Here's how the part is built. I have some questions about the finished solid (model axes, mm). Face numbers are marked on the shaded views. Give positions to 0.01 mm unless a question says otherwise; leave off trailing zeros. Order: outer loops, then holes, each group sorted by start corner. A loop starts at its lowest first (then second) coordinate and runs counter-clockwise, first axis right, second up. Notation, with made-up numbers: M -19,22 L -5,22 A23 ccw -5,48 Z; hole C -7,80 d4. An arc over 180 degrees is marked long. Use one line per item in the form item = value.
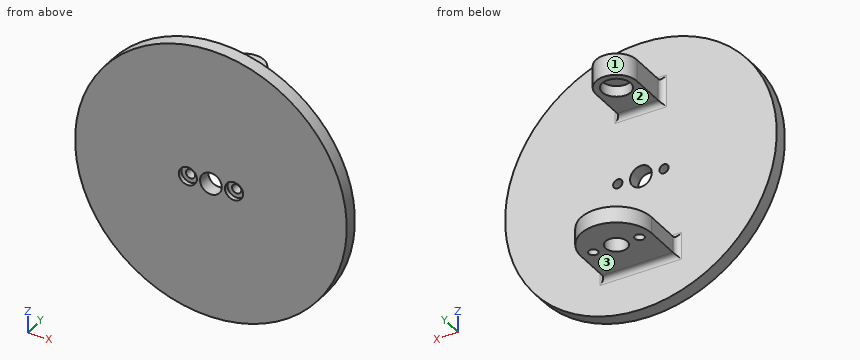
from build123d import *

# Parameters (mm, degrees)
SKETCH1_R                       = 50
SKETCH1_R_2                     = 4
BOSS_EXTRUDE1_DEPTH             = 5
BOSS_EXTRUDE4_DEPTH             = 6
BOSS_EXTRUDE5_DEPTH             = 8
CBORE_FOR_M3_SBHCS1_D           = 3.4
CBORE_FOR_M3_SBHCS1_CBORE_D     = 6.7
CBORE_FOR_M3_SBHCS1_CBORE_DEPTH = 1.65
CBORE_START                     = -29.65
CBORE_FOR_M3_SBHCS2_OUTLINE_R   = 3.35
CBORE_FOR_M3_SBHCS2_DEPTH       = 1.65
CBORE_START_2                   = -34
CBORE_FOR_M3_SBHCS2_2_OUTLINE_R = 1.7
CBORE_FOR_M3_SBHCS2_2_DEPTH     = 4.35
SKETCH29_R                      = 4
CUT_EXTRUDE1_DEPTH              = 6
SKETCH30_R                      = 5.25
CUT_EXTRUDE2_DEPTH              = 4
FILLET1_R                       = 2


# Read off the part's stored shape, not the designer's step: CBORE for M3 SBHCS2
with BuildPart() as part:
    # Sketch1 → Boss-Extrude1 (new body)
    with BuildSketch(Plane(origin=(0, 0, 0), x_dir=(1, 0, 0), z_dir=(0, 1, 0))):
        with Locations(Location((0, 0, 0), (0, 0, 270))):
            Circle(SKETCH1_R)
        with Locations(Location((0, 0, 0), (0, 0, 270))):
            Circle(SKETCH1_R_2, mode=Mode.SUBTRACT)
    extrude(amount=BOSS_EXTRUDE1_DEPTH)

    # Sketch2 → Boss-Extrude4 (add)
    with BuildSketch(Plane.XY.offset(-28)):
        with BuildLine():
            Line((-13, 5), (-13, 20))
            ThreePointArc((-13, 20), (0, 33), (13, 20))
            Line((13, 20), (13, 5))
            Line((13, 5), (-13, 5))
        make_face()
    extrude(amount=-BOSS_EXTRUDE4_DEPTH)

    # Sketch24 → Boss-Extrude5 (add)
    with BuildSketch(Plane.XY.offset(33)):
        with BuildLine():
            Line((-7.5, 5), (-7.5, 20))
            ThreePointArc((-7.5, 20), (0, 27.5), (7.5, 20))
            Line((7.5, 20), (7.5, 5))
            Line((7.5, 5), (-7.5, 5))
        make_face()
    extrude(amount=-BOSS_EXTRUDE5_DEPTH)

    # CBORE for M3 SBHCS1 (through all)
    with Locations(Plane(origin=(0, 0, 0), x_dir=(-1, 0, 0), z_dir=(0, -1, 0))):
        with Locations((-8.5, 0), (8.5, 0)):
            CounterBoreHole(CBORE_FOR_M3_SBHCS1_D / 2, CBORE_FOR_M3_SBHCS1_CBORE_D / 2, CBORE_FOR_M3_SBHCS1_CBORE_DEPTH)

    # CBORE for M3 SBHCS2 outline → CBORE for M3 SBHCS2 (cut)
    with BuildSketch(Plane.XY.offset(CBORE_START)):
        with Locations((-8.5, 20)):
            Circle(CBORE_FOR_M3_SBHCS2_OUTLINE_R)
        with Locations((8.5, 20)):
            Circle(CBORE_FOR_M3_SBHCS2_OUTLINE_R)
    extrude(amount=CBORE_FOR_M3_SBHCS2_DEPTH, mode=Mode.SUBTRACT)

    # CBORE for M3 SBHCS2 2 outline → CBORE for M3 SBHCS2 2 (cut)
    with BuildSketch(Plane.XY.offset(CBORE_START_2)):
        with Locations((-8.5, 20)):
            Circle(CBORE_FOR_M3_SBHCS2_2_OUTLINE_R)
        with Locations((8.5, 20)):
            Circle(CBORE_FOR_M3_SBHCS2_2_OUTLINE_R)
    extrude(amount=CBORE_FOR_M3_SBHCS2_2_DEPTH, mode=Mode.SUBTRACT)

    # Sketch29 → Cut-Extrude1 (cut)
    with BuildSketch(Plane.XY.offset(-28)):
        with Locations((0, 20)):
            Circle(SKETCH29_R)
    extrude(amount=-CUT_EXTRUDE1_DEPTH, mode=Mode.SUBTRACT)

    # Sketch30 → Cut-Extrude2 (cut)
    with BuildSketch(Plane(origin=(0, 0, 25), x_dir=(-1, 0, 0), z_dir=(0, 0, -1))):
        with Locations((0, 19.924351103)):
            Circle(SKETCH30_R)
    extrude(amount=-CUT_EXTRUDE2_DEPTH, mode=Mode.SUBTRACT)

    # Fillet1
    fillet1_edges = [part.edges().sort_by_distance(p)[0] for p in [
        (0, 5, -34),
        (13, 5, -31),
        (-13, 5, -31),
        (0, 5, -28),
        (0, 5, 25),
        (7.5, 5, 29),
        (-7.5, 5, 29),
        (0, 5, 33),
    ]]
    fillet(fillet1_edges, radius=FILLET1_R)


solid = part.part
Q1. I want a section at C-C on x = 0. Write out the boundary of the cut face in (y, z).
Found:
outline = M 0,-50 L 5,-50 L 5,-36 A2 cw 7,-34 L 16,-34 L 16,-28 L 7,-28 A2 cw 5,-26 L 5,-4 L 0,-4 Z; M 0,4 L 5,4 L 5,23 A2 cw 7,25 L 14.67,25 L 14.67,29 L 25.17,29 L 25.17,25 L 27.5,25 L 27.5,33 L 7,33 A2 cw 5,35 L 5,50 L 0,50 Z; M 24,-34 L 33,-34 L 33,-28 L 24,-28 Z
Q2. I want a section at D-D on z = 20.5. Write out the boundary of the cut face in (x, y), then the cut area to 3 significant figures.
Found:
outline = M -45.6,0 L 45.6,0 L 45.6,5 L -45.6,5 Z
area = 456 mm²
Q3. I want a section at B-B on y = 10.5. Write out the boundary of the cut face in (x, z).
Found:
outline = M -13,-34 L 13,-34 L 13,-28 L -13,-28 Z; M -7.5,25 L 7.5,25 L 7.5,33 L -7.5,33 Z
Q4. I need wall thicknesses on L1, parallel to Z at x = 1, y = 26.5; L2, parallel to X at y = 16.5, z = 31; L3, parallel to Y at x = -10, z = 8.5. Which ranges of each line are inside material? Lowest first, please.
Found:
L1 = -34 to -28, 25 to 33
L2 = -7.5 to 7.5
L3 = 0 to 5
Q5. I'm going to push flat-ended pins straight in: pin 1 Ø1 at (x, z) = (-35, -16) entering from +Y; pin 2 Ø3.5 at (x, y) = (-7.5, 20.5) entering from +Z; pin 3 Ø10.5 at (x, y) = (8.5, 20) entering from -Z; pin 4 Ø1.5 at (y, z) = (6, 2.5) entering from +X. Where does each tip first touch, or does it pass through?
Found:
pin_1 = 5
pin_2 = 33
pin_3 = -34
pin_4 = through
Q6. Thinking about a two-plate mould opening in Z: for the marked faces 1, 2 and 3, which applies, +Z half, -Z half, draft (parallel to the pull), parting line (faces both ways), or undercut?
Found:
face_1 = draft
face_2 = undercut
face_3 = -Z half
Q7. I want a section at A-A on z = 0. Write out the boundary of the cut face in (x, y), then the cut area to 3 significant figures.
Found:
outline = M -50,0 L -11.85,0 L -11.85,1.65 L -10.2,1.65 L -10.2,5 L -50,5 Z; M -6.8,1.65 L -5.15,1.65 L -5.15,0 L -4,0 L -4,5 L -6.8,5 Z; M 4,0 L 5.15,0 L 5.15,1.65 L 6.8,1.65 L 6.8,5 L 4,5 Z; M 10.2,1.65 L 11.85,1.65 L 11.85,0 L 50,0 L 50,5 L 10.2,5 Z
area = 415 mm²
